```python
from build123d import *

# Parameters (mm, degrees)
BOX001_W     = 45
BOX001_H     = 57
BOX001_DEPTH = 11
BOX_W        = 48
BOX_H        = 60
BOX_DEPTH    = 10
FILLET004_R  = 4
FILLET005_R  = 4
FILLET006_R  = 4
FILLET007_R  = 3
FILLET008_R  = 2


with BuildPart() as box001:
    # Box001 → Box001 (new body)
    with BuildSketch(Plane(origin=(-2, -2, 46), x_dir=(1, 0, 0), z_dir=(0, 0, 1))):
        with Locations((22.5, 28.5)):
            Rectangle(BOX001_W, BOX001_H)
    extrude(amount=BOX001_DEPTH)


with BuildPart() as tapa001:
    # Box → Box (new body)
    with BuildSketch(Plane(origin=(-4, -4, 50), x_dir=(1, 0, 0), z_dir=(0, 0, 1))):
        with Locations((24, 30)):
            Rectangle(BOX_W, BOX_H)
    extrude(amount=BOX_DEPTH)

    # Cut: cut Box001
    add(box001.part, mode=Mode.SUBTRACT)

    # Fillet004
    fillet004_edges = [tapa001.edges().sort_by_distance(p)[0] for p in [
        (44, -4, 55),
    ]]
    fillet(fillet004_edges, radius=FILLET004_R)

    # Fillet005
    fillet005_edges = [tapa001.edges().sort_by_distance(p)[0] for p in [
        (-4, -4, 55),
    ]]
    fillet(fillet005_edges, radius=FILLET005_R)

    # Fillet006
    fillet006_edges = [tapa001.edges().sort_by_distance(p)[0] for p in [
        (-4, 56, 55),
    ]]
    fillet(fillet006_edges, radius=FILLET006_R)

    # Fillet007
    fillet007_edges = [tapa001.edges().sort_by_distance(p)[0] for p in [
        (44, 56, 55),
    ]]
    fillet(fillet007_edges, radius=FILLET007_R)

    # Fillet008
    fillet008_edges = [tapa001.edges().sort_by_distance(p)[0] for p in [
        (44, 26.5, 60),
    ]]
    fillet(fillet008_edges, radius=FILLET008_R)


solid = tapa001.part
```
Input: part model. Units: mm. Frame: model coordinates. A direction names the side the tool comes from. Give positions to 0.01 mm unless a question says otherwise; leave off trailing zeros. Write each loop counter-clockwise with the first axis right and the second up, starting at its lowest first coordinate (ties: lowest second). Pieces come first, ordered by that corner, then holes. Notation, with made-up numbers: (-30, -16) - (11, -16) arc R15 ccw to (11, -3) - close; hole circle Ø6 at (73.25, -40). An arc over 180 degrees is marked (long way). Write item = value, one per line. Start each with the question number.
1. Section query C-C, the plane x = 28. Output: boundary loops of the cut face in (y, z).
2. Mould query, pull axis X, two halves, no side actions, for faces 3 (the flat face through (-4, 26, 54)), 4 (the cylindrical face through (42.797, -2.859, 54.056)), 5 (the flat face through (-2, 26, 53)), 6 (the cylindrical face through (20.28, -3.43, 59.4)). Classes: released by +X, released by -X, zero draft, split by the parting line, or undercut.
3. Ray query, L1, parallel to Y at x = 11.5, z = 55.5; L2, parallel to X at y = 23.5, z = 56.5; L3, parallel to Z at x = 31.5, y = 33.5. Return the intervals inside material, ascending.
4. Section query A-A, the plane z = 54. Output: boundary loops of the cut face in (x, y), then the cut area to 3 significant figures.
5. Access query for faces 1 (the flat face through (43, 26, 53)), 2 (the flat face through (20, -4, 54)). Directions: +Z, -Z, +X, -X, +Y, -Y. A direction counts if a zero-diameter tool reaches every point of the face in a straight line with its end or side. Return the directions, or none.
6. Section query B-B, the plane y = 26.5. Output: boundary loops of the cut face in (x, z), then the cut area to 3 significant figures.
7. First-contact query: pin 1 Ø5 at (x, y) = (27.5, 28) entering from -Z. Flat tip, straight axial feed; report the tip coordinate or a pass-through.
Check sheet entries:
q1.outline = (-4, 50) - (-2, 50) - (-2, 57) - (55, 57) - (55, 50) - (56, 50) - (56, 58) arc R2 ccw to (54, 60) - (-2, 60) arc R2 ccw to (-4, 58) - close
q2.face_3 = released by -X
q2.face_4 = released by +X
q2.face_5 = undercut
q2.face_6 = zero draft
q3.L1 = -4 to -2, 55 to 56
q3.L2 = -4 to -2, 43 to 44
q3.L3 = 57 to 60
q4.outline = (-4, 0) arc R4 ccw to (0, -4) - (40, -4) arc R4 ccw to (44, 0) - (44, 53) arc R3 ccw to (41, 56) - (0, 56) arc R4 ccw to (-4, 52) - close; hole (-2, -2) - (43, -2) - (43, 55) - (-2, 55) - close
q4.area = 303 mm2
q5.face_1 = -Z
q5.face_2 = +Z, -Z, +X, -X, -Y
q6.outline = (-4, 50) - (-2, 50) - (-2, 57) - (43, 57) - (43, 50) - (44, 50) - (44, 58) arc R2 ccw to (42, 60) - (-2, 60) arc R2 ccw to (-4, 58) - close
q6.area = 163 mm2
q7.pin_1 = 57
